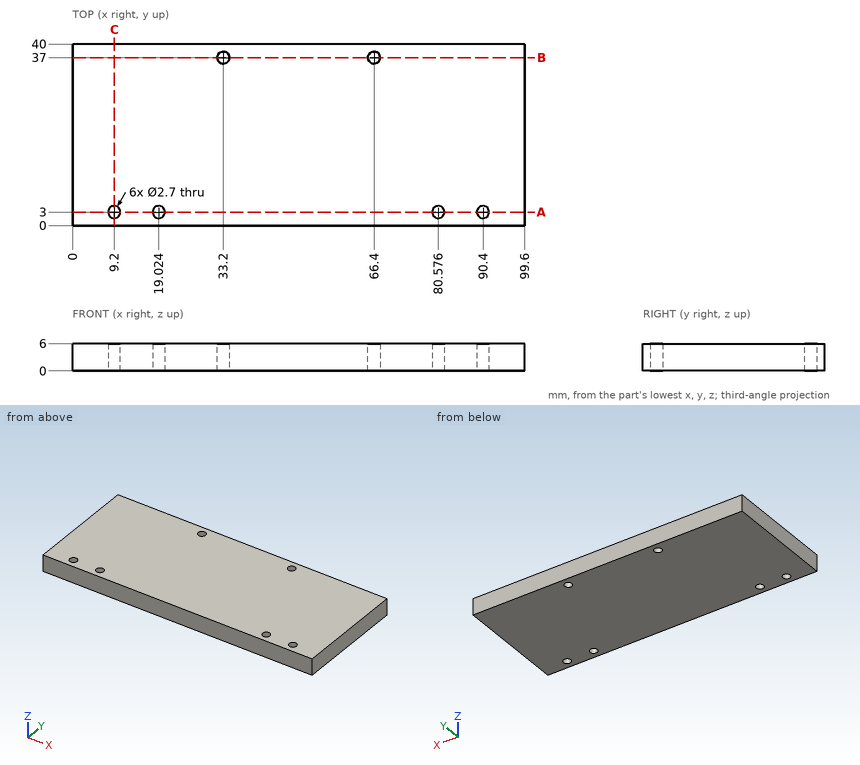
Job drawing, mm, ordinate dimensions from the low corner. One solid piece. Give positions to 0.01 mm unless a question says otherwise; leave off trailing zeros. Order: outer loops, then holes, each group sorted by start corner. A loop starts at its lowest first (then second) coordinate and runs counter-clockwise, first axis right, second up. Notation, with made-up numbers: M -14,4 L -2,4 A13 ccw -2,26 Z; hole C -24,55 d7. An arc over 180 degrees is marked long. Put each result on its own line as item: value. Start each with the question number.
(1) Band-saw the part on A-A on y = 3. Count the separate pieces of the cut face and the enclosed holes in it, then the cut area to 3 significant figures.
(2) Drill centre line: L1, parallel to Y at x = 66.4, z = 4.3. Where is it in solid material? Low to high. Write a range as [from, to].
(3) Band-saw the part on C-C on x = 9.2. Give the cut face in (y, z).
(4) Pin check, flat tip, straight feed: pin 1 Ø1.6 at (x, y) = (90.4, 3) entering from +Z. Stop position of the tip, or through.
(5) Band-saw the part on B-B on y = 37. Give the cut face in (x, z).
Results below:
1. separate pieces: 5
1. enclosed holes: 0
1. area: 533 mm2
2. L1: y = [0, 35.65], [38.35, 40]
3. outline: M 0,0 L 1.65,0 L 1.65,6 L 0,6 Z; M 4.35,0 L 40,0 L 40,6 L 4.35,6 Z
4. pin 1: passes through
5. outline: M 0,0 L 31.85,0 L 31.85,6 L 0,6 Z; M 34.55,0 L 65.05,0 L 65.05,6 L 34.55,6 Z; M 67.75,0 L 99.6,0 L 99.6,6 L 67.75,6 Z
